```python
from build123d import *

# Parameters (mm, degrees)
SKETCH1_W               = 101.6
SKETCH1_H               = 76.2
BOSS_EXTRUDE1_DEPTH     = 19.05
F_1_4_20_TAPPED_HOLE1_D = 5.1054
LPATTERN1_COUNT         = 4
LPATTERN1_PITCH         = 25.4
LPATTERN1_COUNT_DIR2    = 3
LPATTERN1_PITCH_DIR2    = 25.4


with BuildPart() as part:
    # Sketch1 → Boss-Extrude1 (new body)
    with BuildSketch(Plane.XY):
        with Locations((50.8, 38.1)):
            Rectangle(SKETCH1_W, SKETCH1_H)
    extrude(amount=BOSS_EXTRUDE1_DEPTH)

    # 1/4-20 Tapped Hole1 (through all)
    with Locations(Plane.XY.offset(19.05)):
        with Locations((12.7, 63.5)):
            f_1_4_20_tapped_hole1 = Hole(F_1_4_20_TAPPED_HOLE1_D / 2)

    # LPattern1: 1_4-20 Tapped Hole1 4 × 3
    with Locations(*[(i * LPATTERN1_PITCH, -j * LPATTERN1_PITCH_DIR2, 0) for i in range(LPATTERN1_COUNT) for j in range(LPATTERN1_COUNT_DIR2) if (i, j) != (0, 0)]):
        add(f_1_4_20_tapped_hole1, mode=Mode.SUBTRACT)


solid = part.part
```
Geometry check sheet. Reference: the model listing, model coordinates, mm. Round coordinates to 2 decimals unless told otherwise and drop trailing zeros. Loops run counter-clockwise (first coordinate to the right, second up) from the corner with the lowest first, then second, coordinate; pieces in that order, holes last. Notation, with made-up numbers: M 46,68 L 68,68 A26 cw 68,102 Z; hole C -16.5,35.5 d11. An arc over 180 degrees is marked long. Return JSON: item names as keys, results as strings. Group by question number.
(1) Section check A-A, the plane y = 12.7. Enter the section's corners in (x, z), and give its area (3 significant figures).
(2) Section check D-D, the plane x = 88.5. Enter the section's corners in (y, z), and give its area (3 significant figures).
(3) Section check C-C, the plane x = 38.1. Enter the section's corners in (y, z), and give its area (3 significant figures).
(4) Mould release check, pull along Y, two halves, no side actions. Record for faces 1 (the face through (50, 39, 0)), 2 (the face through (10.265, 13.467, 9.392)), 3 (the face through (50, 0, 9)): pulls with the +Y half, pulls with the -Y half, needs draft (parallel to the pull), parting line crosses it, or undercut.
(5) Scan lines: line 1 along Y through (x, z) = (12.7, 11); line 2 along X through (y, z) = (38, 3.75); line 3 along Y through (x, z) = (89.5, 6.5). Record each from-to range of solid material in increasing order. Write a range as [from, to].
(6) Section check B-B, the plane z = 17.25. Give the number of separate pieces and of enclosed holes in the cut face, and give its area (3 significant figures).
Data:
{
 "1": {"outline": "M 0,0 L 10.15,0 L 10.15,19.05 L 0,19.05 Z; M 15.25,0 L 35.55,0 L 35.55,19.05 L 15.25,19.05 Z; M 40.65,0 L 60.95,0 L 60.95,19.05 L 40.65,19.05 Z; M 66.05,0 L 86.35,0 L 86.35,19.05 L 66.05,19.05 Z; M 91.45,0 L 101.6,0 L 101.6,19.05 L 91.45,19.05 Z", "area": "1,550 mm²"},
 "2": {"outline": "M 0,0 L 10.18,0 L 10.18,19.05 L 0,19.05 Z; M 15.22,0 L 35.58,0 L 35.58,19.05 L 15.22,19.05 Z; M 40.62,0 L 60.98,0 L 60.98,19.05 L 40.62,19.05 Z; M 66.02,0 L 76.2,0 L 76.2,19.05 L 66.02,19.05 Z", "area": "1,160 mm²"},
 "3": {"outline": "M 0,0 L 10.15,0 L 10.15,19.05 L 0,19.05 Z; M 15.25,0 L 35.55,0 L 35.55,19.05 L 15.25,19.05 Z; M 40.65,0 L 60.95,0 L 60.95,19.05 L 40.65,19.05 Z; M 66.05,0 L 76.2,0 L 76.2,19.05 L 66.05,19.05 Z", "area": "1,160 mm²"},
 "4": {"face 1": "needs draft", "face 2": "undercut", "face 3": "pulls with the -Y half"},
 "5": {"line 1": "[0, 10.15], [15.25, 35.55], [40.65, 60.95], [66.05, 76.2]", "line 2": "[0, 10.15], [15.25, 35.55], [40.65, 60.95], [66.05, 86.35], [91.45, 101.6]", "line 3": "[0, 10.22], [15.18, 35.62], [40.58, 61.02], [65.98, 76.2]"},
 "6": {"separate pieces": "1", "enclosed holes": "12", "area": "7,500 mm²"}
}
